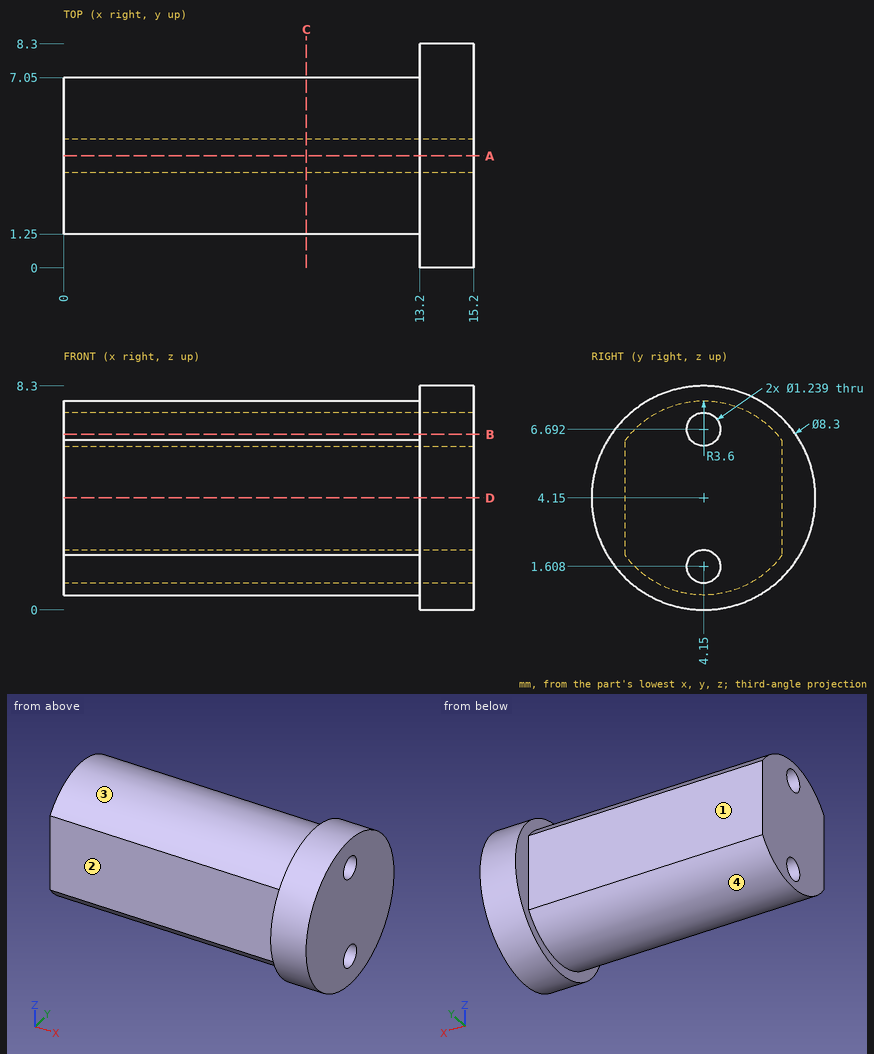
Check sheet for the drawn part. Datum: minimum x, y, z corner. Units: mm. A direction names the side the tool comes from. Round coordinates to 2 decimals unless told otherwise and drop trailing zeros. Loops run counter-clockwise (first coordinate to the right, second up) from the corner with the lowest first, then second, coordinate; pieces in that order, holes last.
Item 1: Cross-section at A-A on y = 4.15. Record the boundary of the cut face in (x, z).
Item 2: Cross-section at D-D on z = 4.15. Record the boundary of the cut face in (x, y).
Item 3: Thickness scan on line 1 (Z direction, x = 4, y = 4); line 2 (X direction, y = 7.25, z = 4.75); line 3 (Z direction, x = 2, y = 4.5) (1 decimal). Record the ranges inside material, lowest first.
Item 4: Gauge pin test, flat ends, axial feed: pin 1 (3.5 mm diameter, centred on x = 4, z = 4, fed in from -Y); pin 2 (4.5 mm diameter, centred on x = 8, z = 4.5, fed in from +Y); pin 3 (1 mm diameter, centred on y = 4.15, z = 1.61, fed in from +X); pin 4 (2 mm diameter, centred on x = 10.5, y = 3.5, fed in from +Z). Record the tip position at first contact, or that the pin passes through.
Item 5: Cross-section at C-C on x = 9. Record the boundary of the cut face in (y, z).
Item 6: Cross-section at B-B on z = 6.5. Record the boundary of the cut face in (x, y).
Item 7: Access from +Z, -Z, +X, -X, +Y, -Y to the whole of each face (thin tool, end or side, straight path). Record for the marked faces 1, 2, 3 and 4.
Answer sheet:
1. outline: (0, 0.55) - (13.2, 0.55) - (13.2, 0) - (15.2, 0) - (15.2, 0.99) - (0, 0.99) - close; (0, 2.23) - (15.2, 2.23) - (15.2, 6.07) - (0, 6.07) - close; (0, 7.31) - (15.2, 7.31) - (15.2, 8.3) - (13.2, 8.3) - (13.2, 7.75) - (0, 7.75) - close
2. outline: (0, 1.25) - (13.2, 1.25) - (13.2, 0) - (15.2, 0) - (15.2, 8.3) - (13.2, 8.3) - (13.2, 7.05) - (0, 7.05) - close
3. line 1: z = 0.55 to 1.01, 2.21 to 6.09, 7.29 to 7.75
3. line 2: x = 13.2 to 15.2
3. line 3: z = 0.6 to 1.1, 2.1 to 6.2, 7.2 to 7.7
4. pin 1: stops at y = 1.25
4. pin 2: stops at y = 7.05
4. pin 3: passes through
4. pin 4: stops at z = 7.75
5. outline: (1.25, 2.02) arc R3.6 ccw to (7.05, 2.02) - (7.05, 6.28) arc R3.6 ccw to (1.25, 6.28) - close; hole circle Ø1.24 at (4.15, 1.61); hole circle Ø1.24 at (4.15, 6.69)
6. outline: (0, 1.42) - (13.2, 1.42) - (13.2, 0.73) - (15.2, 0.73) - (15.2, 3.56) - (0, 3.56) - close; (0, 4.74) - (15.2, 4.74) - (15.2, 7.57) - (13.2, 7.57) - (13.2, 6.88) - (0, 6.88) - close
7. face 1: +Z, -Z, -X, +Y
7. face 2: +Z, -Z, -X, -Y
7. face 3: +Z, -X
7. face 4: -Z, -X
